from build123d import *

# Parameters (mm, degrees)
BOSS_EXTRUDE1_DEPTH = 5
FILLET2_R           = 1


with BuildPart() as part:
    # Sketch1 → Boss-Extrude1 (new body)
    with BuildSketch(Plane.XY):
        with BuildLine():
            Line((-9.132007365, 0), (-9.132007365, 12))
            ThreePointArc((-9.132007365, 12), (-3.960686979, 17.171320386), (1.210633407, 12))
            Line((1.210633407, 12), (1.210633407, 0))
            Line((1.210633407, 0), (-9.132007365, 0))
        make_face()
    extrude(amount=BOSS_EXTRUDE1_DEPTH)

    # Fillet2
    fillet2_edges = [part.edges().sort_by_distance(p)[0] for p in [
        (-3.960686979, 17.171320386, 5),
        (-9.132007365, 6, 5),
        (-3.960686979, 0, 5),
        (-9.132007365, 6, 0),
        (-3.960686979, 17.171320386, 0),
        (1.210633407, 6, 0),
        (-3.960686979, 0, 0),
        (1.210633407, 6, 5),
        (-9.132007365, 0, 2.5),
        (1.210633407, 0, 2.5),
    ]]
    fillet(fillet2_edges, radius=FILLET2_R)


solid = part.part
Geometry: final body of the model. Coordinates: model frame, mm. Coordinates: 2 decimals unless noted, no trailing zeros. Order: outer loops, then holes, each group sorted by start corner. A loop starts at its lowest first (then second) coordinate and runs counter-clockwise, first axis right, second up.
1) Section A-A (y = 5). Return loops of the section in (x, z).
Result sheet:
outline: (-9.13, 1) arc R1 ccw to (-8.13, 0) - (0.21, 0) arc R1 ccw to (1.21, 1) - (1.21, 4) arc R1 ccw to (0.21, 5) - (-8.13, 5) arc R1 ccw to (-9.13, 4) - close
2) Section C-C (z = 0.55). Return loops of the section in (x, y).
Result sheet:
outline: (-9.03, 1) arc R0.89 ccw to (-8.13, 0.11) - (0.21, 0.11) arc R0.89 ccw to (1.1, 1) - (1.1, 12) arc R5.06 ccw to (-9.03, 12) - close
3) Ray query, probe 1 along Y at (x, z) = (-7.25, 4); probe 2 along X at (y, z) = (3, 0.8); probe 3 along Y at (x, z) = (-2.75, 0.5). Return the intervals inside material, ascending.
Result sheet:
probe 1: y = 0 to 15.99
probe 2: x = -9.11 to 1.19
probe 3: y = 0.13 to 16.89
4) Section B-B (z = 1.85). Return loops of the section in (x, y), then the cut area to 3 significant figures.
Result sheet:
outline: (-9.13, 1) arc R1 ccw to (-8.13, 0) - (0.21, 0) arc R1 ccw to (1.21, 1) - (1.21, 12) arc R5.17 ccw to (-9.13, 12) - close
area: 166 mm2
